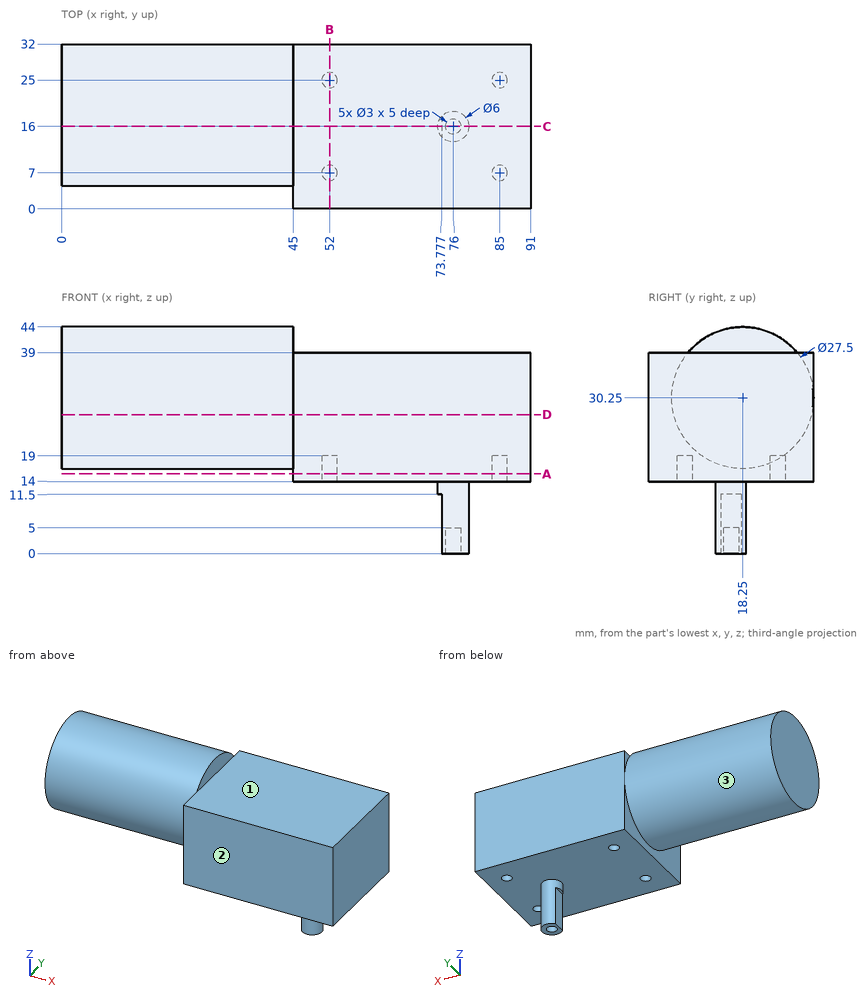
The figure shows three views and two pictorial views of one solid part (mm, origin at its lowest corner). Answer the questions. A direction names the side the tool comes from. Give positions to 0.01 mm unless a question says otherwise; leave off trailing zeros. Write each loop counter-clockwise with the first axis right and the second up, starting at its lowest first coordinate (ties: lowest second). Pieces come first, ordered by that corner, then holes.
Q1. The part is cut by section B-B on x = 52. Give the vertices of the cut face in (y, z), and give its area (3 significant figures).
Answer:
outline: (0, 14) - (5.5, 14) - (5.5, 19) - (8.5, 19) - (8.5, 14) - (23.5, 14) - (23.5, 19) - (26.5, 19) - (26.5, 14) - (32, 14) - (32, 39) - (0, 39) - close
area: 770 mm2
Q2. The part is cut by section C-C on y = 16. Give the vertices of the cut face in (x, z), and give its area (3 significant figures).
Answer:
outline: (0, 16.69) - (45, 16.69) - (45, 14) - (73, 14) - (73, 11.5) - (73.78, 11.5) - (73.78, 0) - (74.5, 0) - (74.5, 5) - (77.5, 5) - (77.5, 0) - (79, 0) - (79, 14) - (91, 14) - (91, 39) - (45, 39) - (45, 43.81) - (0, 43.81) - close
area: 2,430 mm2
Q3. Given pin 1 (2.5 mm diameter, centred on x = 52, y = 25, fed in from +Z); pin 2 (1.5 mm diameter, centred on x = 51.5, y = 25.5, fed in from -Z); pin 3 (4 mm diameter, centred on y = 20, z = 41.5, fed in from +X), each flat-ended and moving along its own axis, determine where each tip first touches the part or whether it passes through.
Answer:
pin 1: stops at z = 39
pin 2: stops at z = 19
pin 3: stops at x = 45
Q4. The part is cut by section D-D on z = 27. Give the vertices of the cut face in (x, y), and give its area (3 significant figures).
Answer:
outline: (0, 4.89) - (45, 4.89) - (45, 0) - (91, 0) - (91, 32) - (45, 32) - (45, 31.61) - (0, 31.61) - close
area: 2,670 mm2
Q5. A tool of negligible diameter and unlimited length cuts with its end or side. For the marked faces 1, 2 and 3, from which of +Z, -Z, +X, -X, +Y, -Y can it reach the whole face along a straight path? Write none if from no direction.
Answer:
face 1: +Z, +X, +Y, -Y
face 2: +Z, -Z, +X, -X, -Y
face 3: -X
Q6. Straight lines are drawn through the part: L1, parallel to Y at x = 85, z = 17.9; L2, parallel to Y at x = 76, z = 3.4; L3, parallel to X at y = 17.5, z = 40. For each, find the intervals that lie inside material, in ascending order.
Answer:
L1: y = 0 to 5.5, 8.5 to 23.5, 26.5 to 32
L2: y = 13 to 14.5, 17.5 to 19
L3: x = 0 to 45
Q7. The part is cut by section A-A on z = 15.5. Give the vertices of the cut face in (x, y), and give its area (3 significant figures).
Answer:
outline: (45, 0) - (91, 0) - (91, 32) - (45, 32) - close; hole circle Ø3 at (52, 7); hole circle Ø3 at (52, 25); hole circle Ø3 at (85, 7); hole circle Ø3 at (85, 25)
area: 1,440 mm2
